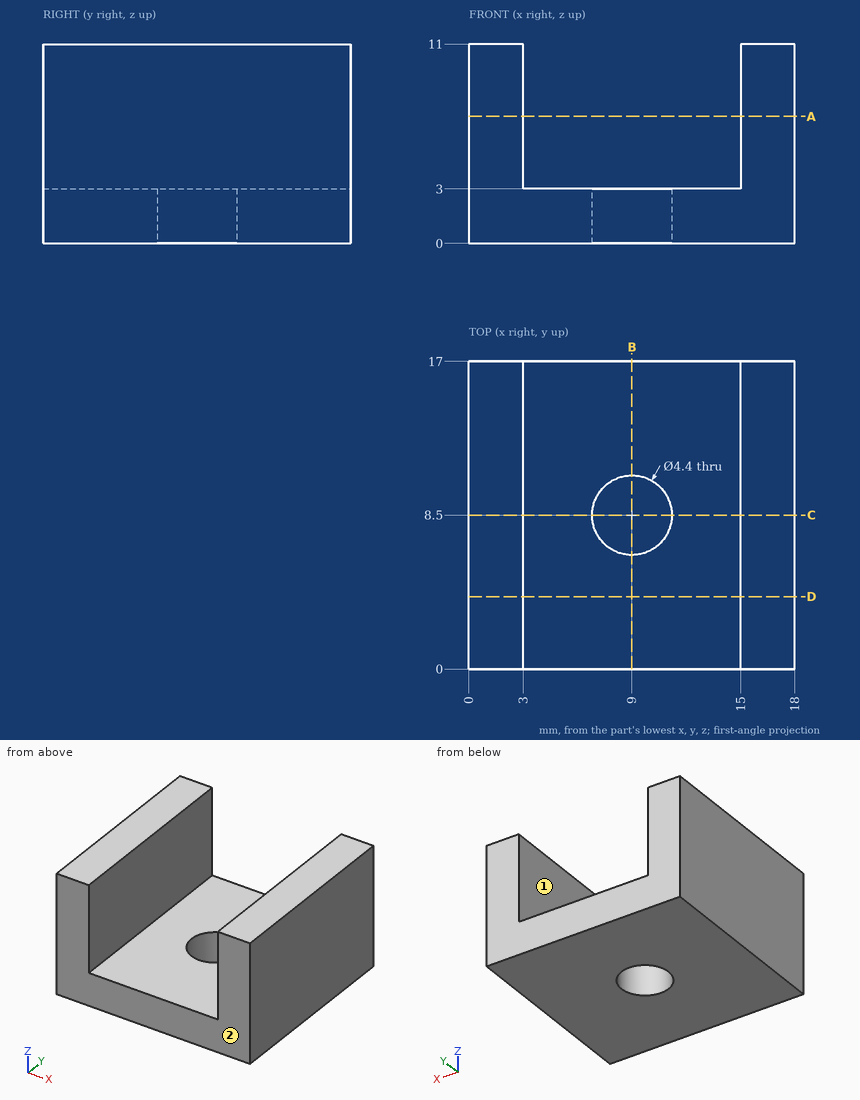
Check sheet for the drawn part. Datum: minimum x, y, z corner. Units: mm. A direction names the side the tool comes from. Give positions to 0.01 mm unless a question says otherwise; leave off trailing zeros. Loops run counter-clockwise (first coordinate to the right, second up) from the corner with the lowest first, then second, coordinate; pieces in that order, holes last.
1) Depth check by flat-ended pin: pin 1 Ø2 at (x, z) = (7, 4.5) entering from +Y; pin 2 Ø3.5 at (x, y) = (10.5, 7.5) entering from +Z. Enter the tip coordinate at first touch or a pass-through.
2) Sectioned sample at D-D, the plane y = 4. Enter the section's corners in (x, z).
3) Sectioned sample at A-A, the plane z = 7. Enter the section's corners in (x, y), then the cut area to 3 significant figures.
4) Sectioned sample at C-C, the plane y = 8.5. Enter the section's corners in (x, z).
5) Sectioned sample at B-B, the plane x = 9. Enter the section's corners in (y, z), then the cut area to 3 significant figures.
6) Thickness scan on line 1 along X through (y, z) = (14, 8); line 2 along Y through (x, z) = (9, 0.65); line 3 along Z through (x, y) = (7.5, 6). Record the ranges inside material, lowest first.
7) Set-up check for the marked faces 1 and 2: record each of +Z, -Z, +X, -X, +Y, -Y from which the full face is reachable in a straight line by a thin tool's end or side.
Answers:
1. pin 1: passes through
1. pin 2: stops at z = 3
2. outline: (0, 0) - (18, 0) - (18, 11) - (15, 11) - (15, 3) - (3, 3) - (3, 11) - (0, 11) - close
3. outline: (0, 0) - (3, 0) - (3, 17) - (0, 17) - close; (15, 0) - (18, 0) - (18, 17) - (15, 17) - close
3. area: 102 mm2
4. outline: (0, 0) - (6.8, 0) - (6.8, 3) - (3, 3) - (3, 11) - (0, 11) - close; (11.2, 0) - (18, 0) - (18, 11) - (15, 11) - (15, 3) - (11.2, 3) - close
5. outline: (0, 0) - (6.3, 0) - (6.3, 3) - (0, 3) - close; (10.7, 0) - (17, 0) - (17, 3) - (10.7, 3) - close
5. area: 37.8 mm2
6. line 1: x = 0 to 3, 15 to 18
6. line 2: y = 0 to 6.3, 10.7 to 17
6. line 3: z = 0 to 3
7. face 1: +Z, +Y, -Y
7. face 2: +Z, -Z, +X, -X, -Y
